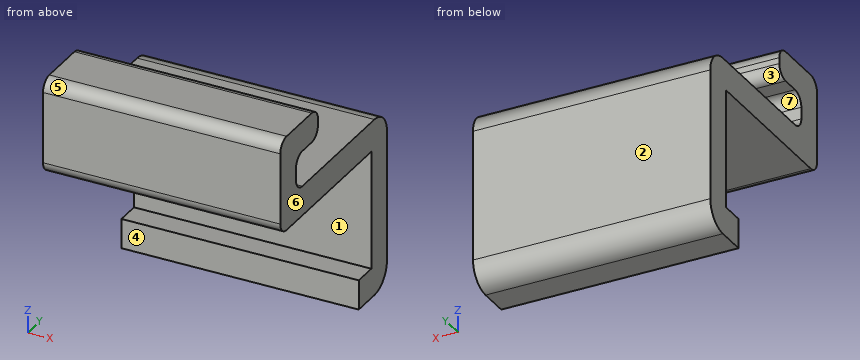
```python
from build123d import *

# Parameters (mm, degrees)
F1_DEPTH = 20
F2_R     = 4
F3_R     = 4
F4_R     = 2


with BuildPart() as f1:
    # F0 (on Right) → F1 (new body, symmetric)
    with BuildSketch(Plane.YZ):
        Polygon((-9.808125, -28.503724), (-13.808125, -28.503724), (-13.808125, -33.503724), (-4.808125, -33.503724), (-4.808125, -3.503724), (-33.808125, -3.503724), (-33.808125, 2.496276), (-26.808125, 2.496276), (-26.808125, 7.496276), (-38.808125, 7.496276), (-38.808125, -8.503724), (-9.808125, -8.503724), align=None)
    extrude(amount=F1_DEPTH, both=True)

    # F2
    f2_edges = [f1.edges().sort_by_distance(p)[0] for p in [
        (0, -4.808125, -3.503724),
    ]]
    fillet(f2_edges, radius=F2_R)

    # F3
    f3_edges = [f1.edges().sort_by_distance(p)[0] for p in [
        (0, -4.808125, -33.503724),
    ]]
    fillet(f3_edges, radius=F3_R)

    # F4
    f4_edges = [f1.edges().sort_by_distance(p)[0] for p in [
        (0, -33.808125, 2.496276),
        (0, -26.808125, 2.496276),
        (0, -26.808125, 7.496276),
        (0, -38.808125, 7.496276),
        (0, -38.808125, -8.503724),
        (0, -33.808125, -3.503724),
    ]]
    fillet(f4_edges, radius=F4_R)


solid = f1.part
```
Could you check a few things on this model? Use its own coordinates, in mm. Face numbers are marked on the shaded views. A direction names the side the tool comes from. Round coordinates to 2 decimals unless told otherwise and drop trailing zeros. Order: outer loops, then holes, each group sorted by start corner. A loop starts at its lowest first (then second) coordinate and runs counter-clockwise, first axis right, second up. Notation, with made-up numbers: (50.25, 88) -> (61.25, 88) arc R25 cw to (61.25, 113) -> close; hole circle Ø9 at (0.5, 85). An arc over 180 degrees is marked (long way). One line per question, with ' | ' between items.
Q1. I'm going to push flat-ended pins straight in: pin 1 (1.1 mm diameter, centred on x = 1, z = 5, fed in from +Y); pin 2 (6 mm diameter, centred on x = -14.5, y = -18.5, fed in from -Z); pin 3 (4.5 mm diameter, centred on x = -8, y = -11.5, fed in from +Z). Where does each tip first touch, or does it pass through?
Computed values:
pin 1: y = -26.81 | pin 2: z = -8.5 | pin 3: z = -3.5
Q2. If we section it at C-C on y = -24.5: Write out the boundary of the cut face in (x, z).
Computed values:
outline: (-20, -8.5) -> (20, -8.5) -> (20, -3.5) -> (-20, -3.5) -> close
Q3. If we section it at B-B on z = -22: Write out the boundary of the cut face in (x, y), plus the area to 3 significant figures.
Computed values:
outline: (-20, -9.81) -> (20, -9.81) -> (20, -4.81) -> (-20, -4.81) -> close | area: 200 mm²
Q4. If I drill on line 1 (Z direction, x = -6, y = -32); line 2 (Z direction, x = 10.5, y = -34); line 3 (Y direction, x = 6, z = -9), over which ranges is the centre line in solid material (lowest first)? Write a range as from..to.
Computed values:
line 1: -8.5..-3.49, 2.49..7.5 | line 2: -8.5..7.5 | line 3: -9.81..-4.81
Q5. Which directions (+Z, -Z, +X, -X, +Y, -Y) give clear straight access to the entire face, cutting with the end or side of a thin tool? Please do the marked faces 1, 2, 3 and 4.
Computed values:
face 1: +X, -X, -Y | face 2: +Z, -Z, +X, -X, +Y | face 3: +X, -X, +Y | face 4: -Z, +X, -X, -Y
Q6. If we section it at A-A on x = 8: Write out the boundary of the cut face in (y, z), plus the area to 3 significant figures.
Computed values:
outline: (-38.81, -6.5) arc R2 ccw to (-36.81, -8.5) -> (-9.81, -8.5) -> (-9.81, -28.5) -> (-13.81, -28.5) -> (-13.81, -33.5) -> (-8.81, -33.5) arc R4 ccw to (-4.81, -29.5) -> (-4.81, -7.5) arc R4 ccw to (-8.81, -3.5) -> (-31.81, -3.5) arc R2 cw to (-33.81, -1.5) -> (-33.81, 0.5) arc R2 cw to (-31.81, 2.5) -> (-28.81, 2.5) arc R2 ccw to (-26.81, 4.5) -> (-26.81, 5.5) arc R2 ccw to (-28.81, 7.5) -> (-36.81, 7.5) arc R2 ccw to (-38.81, 5.5) -> close | area: 396 mm²
Q7. We'd pull the mould along Z, two halves only. Please class the marked faces 5, 6 and 7: released by +Z, released by -Z, zero draft, split by the parting line, or undercut.
Computed values:
face 5: released by +Z | face 6: zero draft | face 7: undercut
